Geometry: final body of the model. Coordinates: model frame, mm. A direction names the side the tool comes from. Round coordinates to 2 decimals unless told otherwise and drop trailing zeros. Write each loop counter-clockwise with the first axis right and the second up, starting at its lowest first coordinate (ties: lowest second). Pieces come first, ordered by that corner, then holes. Notation, with made-up numbers: (36.5, -7.5) -> (86.5, -7.5) arc R21 ccw to (86.5, 12.5) -> close; hole circle Ø1 at (52.25, -37). An arc over 180 degrees is marked (long way). One line per item, written item: value. Start each with the question number.
from build123d import *

# Parameters (mm, degrees)
SKETCH1_R      = 3.175
EXTRUDE1_DEPTH = 1.8542
FILLET1_R      = 1.524
SKETCH2_R      = 1.7526
EXTRUDE2_DEPTH = 12.7
EXTRUDE3_DEPTH = 1.016


with BuildPart() as part:
    # Sketch1 → Extrude1 (new body)
    with BuildSketch(Plane.XY):
        Circle(SKETCH1_R)
    extrude(amount=EXTRUDE1_DEPTH)

    # Fillet1
    fillet1_edges = [part.edges().sort_by_distance(p)[0] for p in [
        (-3.175, 0, 0),
    ]]
    fillet(fillet1_edges, radius=FILLET1_R)

    # Sketch2 → Extrude2 (add)
    with BuildSketch(Plane.XY.offset(1.8542)):
        Circle(SKETCH2_R)
    extrude(amount=EXTRUDE2_DEPTH)

    # Sketch3 → Extrude3 (cut)
    with BuildSketch(Plane(origin=(0, 0, 0), x_dir=(-1, 0, 0), z_dir=(0, 0, -1))):
        Polygon((0.59085384, 0.981566666), (-0.554634748, 1.002477769), (-1.145488588, 0.020911103), (-0.59085384, -0.981566666), (0.554634748, -1.002477769), (1.145488588, -0.020911103), align=None)
    extrude(amount=-EXTRUDE3_DEPTH, mode=Mode.SUBTRACT)


solid = part.part
(1) Pull-direction query (X, two-part tool) for faces 1 (the face through (0.846, 0.519, 0.501)), 2 (the face through (1.67, 0.53, 8.12)), 3 (the face through (0, 0, 14.554)); classes: pulls with the +X half, pulls with the -X half, needs draft (parallel to the pull), parting line crosses it, or undercut.
(2) Section query A-A (z = 7). Output: boundary loops of the cut face in (x, y), and give its area (3 significant figures).
(3) Line query: probe 1 along Z at (x, y) = (0, 0.25); probe 2 along X at (y, z) = (0.25, 13.5); probe 3 along Z at (x, y) = (2, 2). Output: solid intervals per line, ascending.
(4) Set-up query: faces 4 (the face through (-0.69, -3.1, 1.69)), 5 (the face through (1.4, -1.4, 1.854)), 6 (the face through (-0.872, 0.473, 0.501)). Return all of +Z, -Z, +X, -X, +Y, -Y with unobstructed straight access to the full face (end or side cutting, diameter ignored); none if empty.
(5) Pin query (flat end, axial travel): pin 1 (1 mm diameter, centred on y = -1.5, z = 8.5, fed in from -X). Return the tip coordinate at first contact, or that it passes through.
(6) Section query B-B (x = 0). Output: boundary loops of the cut face in (y, z) (3 decimals), and give its area (3 significant figures).
Results list:
1. face 1: undercut
1. face 2: parting line crosses it
1. face 3: needs draft
2. outline: circle Ø3.51 at (0, 0)
2. area: 9.65 mm^2
3. probe 1: z = 1.02 to 14.55
3. probe 2: x = -1.73 to 1.73
3. probe 3: z = 0.56 to 1.85
4. face 4: +Z, -Z
4. face 5: +Z
4. face 6: -Z
5. pin 1: stops at x = -1.44
6. outline: (-3.175, 1.524) arc R1.524 ccw to (-1.651, 0) -> (-0.992, 0) -> (-0.992, 1.016) -> (0.992, 1.016) -> (0.992, 0) -> (1.651, 0) arc R1.524 ccw to (3.175, 1.524) -> (3.175, 1.854) -> (1.753, 1.854) -> (1.753, 14.554) -> (-1.753, 14.554) -> (-1.753, 1.854) -> (-3.175, 1.854) -> close
6. area: 53.3 mm^2
